The listing builds one solid part. Answer for the finished solid, in the listing's coordinates (mm). A direction names the side the tool comes from. Give positions to 0.01 mm unless a question says otherwise; leave off trailing zeros. Order: outer loops, then holes, each group sorted by start corner. A loop starts at its lowest first (then second) coordinate and runs counter-clockwise, first axis right, second up. Notation, with made-up numbers: (5, -20) - (20, -20) arc R27 cw to (20, 19) - close; hole circle Ø4 at (26.25, 9). An arc over 180 degrees is marked (long way). Answer as CSV lines item,"result". Start each with the question number.
1. Which of the six approach directions +Z, -Z, +X, -X, +Y, -Y give full straight-line access (tool end or side, diameter ignored) to faces 1 (the flat face through (1, 6.35, -13)), 2 (the flat face through (-41, -1, -6.35))?
2. Section C-C on z = -10.25 is taken. Give the vertices of the cut face in (x, y) (3 decimals), and give its area (3 significant figures).
3. Flat-ended cylindrical pins translate along their axes: pin 1 (5.5 mm diameter, centred on x = -44.45, y = 0, fed in from -Z); pin 2 (5 mm diameter, centred on x = 43, y = -1, fed in from +Z). Find the tip coordinate at first contact, or state that the pin passes through.
4. Consider line 1 along X through (y, z) = (0, -4.5); line 2 along X through (y, z) = (0, -19.5) (3 decimals); line 3 along Y through (x, z) = (-44.45, -3.25). Determine where each line is inside the solid, lowest interval first. Write a range as [from, to].
5. Section B-B on y = 0 is taken. Count the separate pieces of the cut face and the enclosed holes in it, and give its area (3 significant figures).
6. Determine the mould class of faces 3 (the flat face through (41, 1, -6.35)), 4 (the flat face through (-1, 0, 0)), 5 (the flat face through (-1, -6.35, -13)), 6 (the cylindrical face through (39.73, 0.62, -3.22)) for opening direction Y: +Y half, -Y half, draft (parallel to the pull), parting line (faces both ways), or undercut.
Autodesk Inventor part; units mm, degrees
ref_plane "YZ Plane" through (0, 0, 0) normal (1, 0, 0) x (0, 1, 0)
ref_plane "XZ Plane" through (0, 0, 0) normal (0, 1, 0) x (-1, 0, 0)
ref_plane "XY Plane" through (0, 0, 0) normal (0, 0, 1) x (1, 0, 0)
sketch "Sketch1" plane through (0, 0, 0) normal (0, 0, 1) x (1, 0, 0)
  line L0 (50.8, 6.35) -> (-50.8, 6.35)
  line L1 (-50.8, 6.35) -> (-50.8, -6.35)
  line L2 (-50.8, -6.35) -> (50.8, -6.35)
  line L3 (50.8, -6.35) -> (50.8, 6.35)
  line L4 (50.8, 6.35) -> (-50.8, -6.35) construction
  line L5 (-50.8, 6.35) -> (50.8, -6.35) construction
  point P0 (0, 0)
  dimension "d0" = 101.6
  dimension "d1" = 12.7
extrude "Extrusion1" add sketch "Sketch1" against normal blind 25.4
sketch "Sketch2" plane through (0, 0, 0) normal (0, 0, 1) x (1, 0, 0)
  line L0 (-71.12, 0) -> (71.12, 0)
  line L1 (0, -8.89) -> (0, 8.89)
  line L2 (-50.8, 6.35) -> (-50.8, -6.35)
  line L3 (-50.8, -6.35) -> (50.8, -6.35)
  line L4 (50.8, -6.35) -> (50.8, 6.35)
  line L5 (50.8, 6.35) -> (-50.8, 6.35)
  point P0 (0, 0)
  point P1 (-44.45, 0)
  dimension "d5" = 44.45
hole "Hole1" at (-44.45, 0, 0) direction (0, 0, -1) diameter 6.35 end through all counterbore diameter 9.525 counterbore depth 6.35
mirror "Mirror1" about plane through (0, 0, 0) normal (1, 0, 0) of "Hole1"
equation "\"d11\" = Thickness"
equation "\"BendRadius\" = Thickness"
equation "\"BendReliefWidth\" = Thickness"
equation "\"BendReliefDepth\" = 0.5 * Thickness"
equation "\"CornerReliefSize\" = 4 * Thickness"
equation "\"MinimumRemnant\" = 2 * Thickness"
equation "\"TransitionRadius\" = BendRadius"
equation "\"JacobiRadiusSize\" = BendRadius"
equation "\"GapSize\" = Thickness"
properties part number "3DPrintedFrameBackingPlate"
Checks:
1,face 1,"+Z, -Z, +X, -X, +Y"
1,face 2,"+Z"
2,outline,"(-50.8, -6.35) - (50.8, -6.35) - (50.8, 6.35) - (-50.8, 6.35) - close; hole circle Ø6.35 at (-44.45, 0); hole circle Ø6.35 at (44.45, 0)"
2,area,"1,230 mm²"
3,pin 1,"passes through"
3,pin 2,"stops at z = -6.35"
4,line 1,"x = [-50.8, -49.21], [-39.69, 39.69], [49.21, 50.8]"
4,line 2,"x = [-50.8, -47.625], [-41.275, 41.275], [47.625, 50.8]"
4,line 3,"y = [-6.35, -4.76], [4.76, 6.35]"
5,separate pieces,"3"
5,enclosed holes,"0"
5,area,"2,220 mm²"
6,face 3,"undercut"
6,face 4,"draft"
6,face 5,"-Y half"
6,face 6,"undercut"
